Autodesk Inventor part; units mm, degrees
ref_plane "YZ Plane" through (0, 0, 0) normal (1, 0, 0) x (0, 1, 0)
ref_plane "XZ Plane" through (0, 0, 0) normal (0, 1, 0) x (-1, 0, 0)
ref_plane "XY Plane" through (0, 0, 0) normal (0, 0, 1) x (1, 0, 0)
sketch "Sketch1" plane through (0, 0, 0) normal (0, 1, 0) x (-1, 0, 0)
  circle A0 centre (0, 0) radius 9.75
  circle A1 centre (0, 0) radius 11.25
  dimension "d0" = 19.5
  dimension "d1" = 22.5
extrude "Extrusion1" add sketch "Sketch1" along normal blind 2 contours A0 | A1
sketch "Sketch2" plane through (0, 2, 0) normal (0, 1, 0) x (1, 0, 0)
  circle A0 centre (0, 0) radius 9.75
  dimension "d4" = 19.5
extrude "Extrusion2" cut sketch "Sketch2" against normal blind 1
sketch "Sketch3" plane through (0, 1, 0) normal (0, 1, 0) x (1, 0, 0)
  circle A0 centre (0, 0) radius 8.75
  dimension "d7" = 17.5
extrude "Extrusion3" cut sketch "Sketch3" against normal blind 1
sketch "Sketch4" plane through (0, 0, 0) normal (0, -1, 0) x (1, 0, 0)
  circle A0 centre (0, 0) radius 8.75
  circle A1 centre (0, 0) radius 10.75
  dimension "d10" = 21.5
  dimension "d13" = 17.5
extrude "Extrusion4" add sketch "Sketch4" along normal blind 6
properties part number "685ZZFlanged_Adapter_3mm"
Model file for the job. Use its own axes, mm. A direction names the side the tool comes from. Coordinates: 2 decimals unless noted, no trailing zeros. Loops run counter-clockwise (first coordinate to the right, second up) from the corner with the lowest first, then second, coordinate; pieces in that order, holes last. Notation, with made-up numbers: (27.25, 33.25) - (77.25, 33.25) arc R19 cw to (77.25, 67.25) - close; hole circle Ø9 at (-6.5, -20.75). An arc over 180 degrees is marked (long way). Write item = value, one per line. Start each with the question number.
Item 1: Drop flat-ended pins along their axis: pin 1 Ø1.5 at (y, z) = (0, -5) entering from +X; pin 2 Ø1 at (x, y) = (5.5, -1.5) entering from -Z; pin 3 Ø10.5 at (x, z) = (0, 0) entering from -Y. Give the stop position or say it passes through.
Item 2: Saw through at D-D, the plane y = -2.5. List the corners of the cut face in (x, z).
Item 3: 3-axis set-ups, long thin cutter, end or side, ignore diameter. For faces 4 (the face through (-11, 0, -1)), 5 (the face through (-1.269, 1.507, -9.667)), 6 (the face through (2, -6, -9)): which of +Z, -Z, +X, -X, +Y, -Y reach the whole face in a straight line?
Item 4: Wall check: probe 1 along Z at (x, y) = (0, -0.5); probe 2 along Y at (x, z) = (10, 4.25); probe 3 along Z at (x, y) = (-1.5, 0.75). Give the ranges that are in metal, low to high. Write a range as [from, to].
Item 5: Saw through at C-C, the plane y = 1.5. List the corners of the cut face in (x, z).
Item 6: Saw through at A-A, the plane z = 0. List the corners of the cut face in (x, y).
Item 7: Saw through at B-B, the plane x = 0. List the corners of the cut face in (y, z), then the cut area to 3 significant figures.
Item 8: Pull direction X, two halves, no side cores. Call faces 1 (the face through (-6.944, -2.451, 5.324)), 2 (the face through (-5.19, 0.99, 9.98)), 3 (the face through (0, 2, 10)): +X half, -X half, draft (parallel to the pull), parting line (faces both ways), or undercut.
Answers:
q1.pin_1 = 10.42
q1.pin_2 = -9.52
q1.pin_3 = through
q2.outline = circle Ø21.5 at (0, 0); hole circle Ø17.5 at (0, 0)
q3.face_4 = -Y
q3.face_5 = +Y
q3.face_6 = +Z, -Z, +X, -X, -Y
q4.probe_1 = [-10.75, -8.75], [8.75, 10.75]
q4.probe_2 = [0, 2]
q4.probe_3 = [-11.15, -8.62], [8.62, 11.15]
q5.outline = circle Ø22.5 at (0, 0); hole circle Ø19.5 at (0, 0)
q6.outline = (-11.25, 0) - (-10.75, 0) - (-10.75, -6) - (-8.75, -6) - (-8.75, 1) - (-9.75, 1) - (-9.75, 2) - (-11.25, 2) - close; (8.75, -6) - (10.75, -6) - (10.75, 0) - (11.25, 0) - (11.25, 2) - (9.75, 2) - (9.75, 1) - (8.75, 1) - close
q7.outline = (-6, -10.75) - (0, -10.75) - (0, -11.25) - (2, -11.25) - (2, -9.75) - (1, -9.75) - (1, -8.75) - (-6, -8.75) - close; (-6, 8.75) - (1, 8.75) - (1, 9.75) - (2, 9.75) - (2, 11.25) - (0, 11.25) - (0, 10.75) - (-6, 10.75) - close
q7.area = 32.0 mm2
q8.face_1 = undercut
q8.face_2 = parting line
q8.face_3 = draft
